from build123d import *

# Parameters (mm, degrees)
SKETCH1_R          = 11
EXTRUDE1_DEPTH     = 4
SKETCH3_R          = 8
EXTRUDE3_DEPTH     = 20
SKETCH7_R          = 7.25
CUT_EXTRUDE5_DEPTH = 16
SKETCH4_R          = 6.25
EXTRUDE4_DEPTH     = 14
CHAMFER1_SIZE      = 0.2
CHAMFER3_SIZE      = 0.3
SKETCH5_R          = 10
SKETCH5_R_2        = 8.25
CUT_EXTRUDE1_DEPTH = 1.5
SKETCH6_R          = 0.9
CUT_EXTRUDE2_DEPTH = 5
CHAMFER4_SIZE      = 0.2
SKETCH8_R          = 6
CUT_EXTRUDE6_DEPTH = 2
CHAMFER5_SIZE      = 1
EXTRUDE6_START     = 7.35
SKETCH10_R         = 9.469128054
SKETCH10_R_2       = 8
EXTRUDE6_DEPTH     = 3.5
EXTRUDE5_START     = -7
EXTRUDE5_DEPTH     = 3


with BuildPart() as part:
    # Sketch1 → Extrude1 (new body)
    with BuildSketch(Plane.XY):
        Circle(SKETCH1_R)
    extrude(amount=EXTRUDE1_DEPTH)

    # Sketch3 → Extrude3 (add)
    with BuildSketch(Plane(origin=(0, 0, 0), x_dir=(-1, 0, 0), z_dir=(0, 0, -1))):
        Circle(SKETCH3_R)
    extrude(amount=EXTRUDE3_DEPTH)

    # Sketch7 → Cut-Extrude5 (cut)
    with BuildSketch(Plane.XY.offset(4)):
        Circle(SKETCH7_R)
    extrude(amount=-CUT_EXTRUDE5_DEPTH, mode=Mode.SUBTRACT)

    # Sketch4 → Extrude4 (add)
    with BuildSketch(Plane.XY.offset(-12)):
        Circle(SKETCH4_R)
    extrude(amount=EXTRUDE4_DEPTH)

    # Chamfer1
    chamfer1_edges = [part.edges().sort_by_distance(p)[0] for p in [
        (-6.25, 0, 2),
    ]]
    chamfer(chamfer1_edges, length=CHAMFER1_SIZE)

    # Chamfer3
    chamfer3_edges = [part.edges().sort_by_distance(p)[0] for p in [
        (-11, 0, 4),
    ]]
    chamfer(chamfer3_edges, length=CHAMFER3_SIZE)

    # Sketch5 → Cut-Extrude1 (cut)
    with BuildSketch(Plane(origin=(0, 0, 0), x_dir=(-1, 0, 0), z_dir=(0, 0, -1))):
        Circle(SKETCH5_R)
        Circle(SKETCH5_R_2, mode=Mode.SUBTRACT)
    extrude(amount=-CUT_EXTRUDE1_DEPTH, mode=Mode.SUBTRACT)

    # Sketch6 → Cut-Extrude2 (cut)
    with BuildSketch(Plane.XY.offset(2)):
        with Locations((2.5, 0)):
            Circle(SKETCH6_R)
        with Locations((-2.5, 0)):
            Circle(SKETCH6_R)
    extrude(amount=-CUT_EXTRUDE2_DEPTH, mode=Mode.SUBTRACT)

    # Chamfer4
    chamfer4_edges = [part.edges().sort_by_distance(p)[0] for p in [
        (1.6, 0, 2),
        (-3.4, 0, 2),
    ]]
    chamfer(chamfer4_edges, length=CHAMFER4_SIZE)

    # Sketch8 → Cut-Extrude6 (cut)
    with BuildSketch(Plane(origin=(0, 0, -20), x_dir=(-1, 0, 0), z_dir=(0, 0, -1))):
        Circle(SKETCH8_R)
    extrude(amount=-CUT_EXTRUDE6_DEPTH, mode=Mode.SUBTRACT)

    # Chamfer5
    chamfer5_edges = [part.edges().sort_by_distance(p)[0] for p in [
        (8, 0, -20),
    ]]
    chamfer(chamfer5_edges, length=CHAMFER5_SIZE)

    # Sketch10 → Extrude6 (add)
    with BuildSketch(Plane(origin=(0, 0, 0), x_dir=(-1, 0, 0), z_dir=(0, 0, -1)).offset(EXTRUDE6_START)):
        Circle(SKETCH10_R)
        Circle(SKETCH10_R_2, mode=Mode.SUBTRACT)
    extrude(amount=EXTRUDE6_DEPTH)

    # Sketch9 → Extrude5 (add)
    with BuildSketch(Plane(origin=(0, 0, -18), x_dir=(-1, 0, 0), z_dir=(0, 0, -1)).offset(EXTRUDE5_START)):
        Polygon((-5.484827557, 9.5), (5.484827557, 9.5), (10.969655115, 0), (5.484827557, -9.5), (-5.484827557, -9.5), (-10.969655115, 0), align=None)
    extrude(amount=EXTRUDE5_DEPTH)


solid = part.part
Check sheet for the modelled part. Datum: model origin and axes. Units: mm. A direction names the side the tool comes from. Round coordinates to 2 decimals unless told otherwise and drop trailing zeros. Order: outer loops, then holes, each group sorted by start corner. A loop starts at its lowest first (then second) coordinate and runs counter-clockwise, first axis right, second up. Notation, with made-up numbers: M 49,43 L 65,43 A31 ccw 65,79 Z; hole C 70.25,75 d3. An arc over 180 degrees is marked long. One line per item, written item: value. Start each with the question number.
1. Release check for a two-part mould opening along Z. For faces 1 (the flat face through (0, 0, -18)), 2 (the flat face through (-8.2, 4.8, -12.5)), 3 (the flat face through (3.8, 7.5, 1.5)), 4 (the cylindrical face through (-7.62, -3.16, 0.74)) record: released by +Z, released by -Z, zero draft, split by the parting line, or undercut.
2. Section check B-B on z = -9.75. Enter the section's corners in (x, y), and give its area (3 significant figures).
3. Access from +Z, -Z, +X, -X, +Y, -Y to the whole of each face (thin tool, end or side, straight path). Record for faces 5 (the flat face through (0, 6.5, -11)), 6 (the flat face through (-8.266, -4.684, -12.479)), 7 (the flat face through (2, -8, -11)).
4. Scan lines: line 1 along Z through (x, y) = (-8.5, 2); line 2 along Y through (x, z) = (0, 0.25); line 3 along Y through (x, z) = (-3.75, -6). Record each from-to range of solid material in increasing order.
5. Gauge pin test, flat ends, axial feed: P1, Ø6, axis at y = -7, z = -1, coming from the +X side; P2, Ø1.5, axis at x = 4, z = -8.5, coming from the -Y side; P3, Ø12, axis at x = 6, z = -6.5, coming from the +Y side; P4, Ø9.5, axis at x = -1.5, y = 1, coming from the -Z side. Record the tip position at first contact, or that the pin passes through.
6. Section check A-A on z = -2.25. Enter the section's corners in (x, y).
Results found:
1. face 1: released by -Z
1. face 2: zero draft
1. face 3: undercut
1. face 4: undercut
2. outline: C 0,0 d18.94; C 0,0 d12.5; hole C 0,0 d14.5
2. area: 239 mm^2
3. face 5: +Z
3. face 6: -Z, -X, -Y
3. face 7: none
4. line 1: -14 to -11, -10.85 to -7.35, 1.5 to 4
4. line 2: -11 to -10, -8.25 to -7.25, -6.25 to 6.25, 7.25 to 8.25, 10 to 11
4. line 3: -7.07 to -6.2, -5 to 5, 6.2 to 7.07
5. P1: x = 10.18
5. P2: y = -8.89
5. P3: y = 9.5
5. P4: z = -20
6. outline: C 0,0 d16; C 0,0 d12.5; hole C 0,0 d14.5; hole C -2.5,0 d1.8; hole C 2.5,0 d1.8
